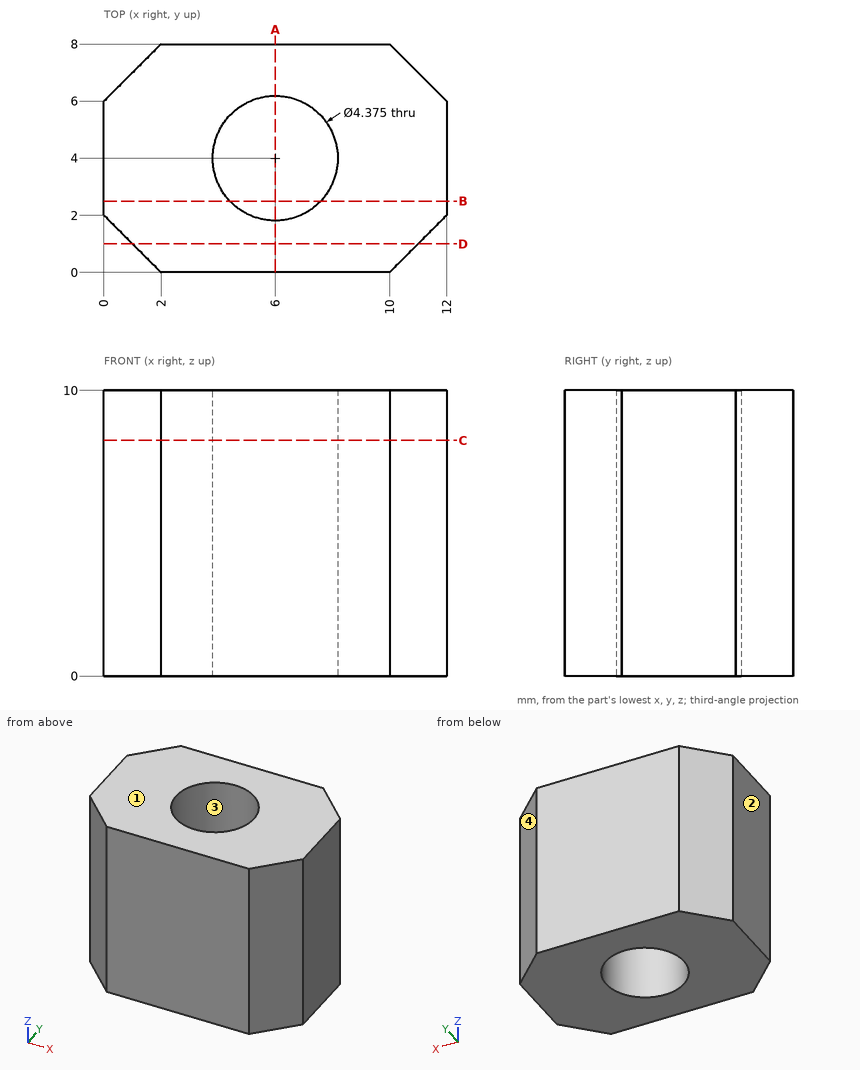
Can you work these out from the drawing? Everything is in mm from the part's minimum corner. Coordinates: 2 decimals unless noted, no trailing zeros. Loops run counter-clockwise (first coordinate to the right, second up) from the corner with the lowest first, then second, coordinate; pieces in that order, holes last.
1. Imagine slicing it at C-C, the plane z = 8.25. Please give me the cut outline in (x, y) (1 decimal), and give its area (3 significant figures).
2. If we mould it in two halves opening along X, with no side actions, what happens to the marked faces 1, 2, 3 and 4? For each: pulls with the +X half, pulls with the -X half, needs draft (parallel to the pull), parting line crosses it, or undercut.
3. Imagine slicing it at A-A, the plane x = 6. Please give me the cut outline in (y, z), and give its area (4 significant figures).
4. Imagine slicing it at D-D, the plane y = 1. Please give me the cut outline in (x, z).
5. I need wall thicknesses on L1, parallel to Y at x = 6, z = 2; L2, parallel to X at y = 3.5, z = 2.25; L3, parallel to Y at x = 7.25, z = 4.25. Which ranges of each line are inside material? Lowest first, please.
6. For P1, Ø4, axis at x = 6, y = 4, coming from the -Z side, with a flat end and sliding along its axis, tell me the tip position at first contact or that it passes through.
7. Imagine slicing it at B-B, the plane y = 2.5. Please give me the cut outline in (x, z).
Taken from the geometry:
1. outline: (0, 2) - (2, 0) - (10, 0) - (12, 2) - (12, 6) - (10, 8) - (2, 8) - (0, 6) - close; hole circle Ø4.4 at (6, 4)
1. area: 73.0 mm2
2. face 1: needs draft
2. face 2: pulls with the -X half
2. face 3: undercut
2. face 4: pulls with the +X half
3. outline: (0, 0) - (1.81, 0) - (1.81, 10) - (0, 10) - close; (6.19, 0) - (8, 0) - (8, 10) - (6.19, 10) - close
3. area: 36.25 mm2
4. outline: (1, 0) - (11, 0) - (11, 10) - (1, 10) - close
5. L1: y = 0 to 1.81, 6.19 to 8
5. L2: x = 0 to 3.87, 8.13 to 12
5. L3: y = 0 to 2.2, 5.8 to 8
6. P1: passes through
7. outline: (0, 0) - (4.41, 0) - (4.41, 10) - (0, 10) - close; (7.59, 0) - (12, 0) - (12, 10) - (7.59, 10) - close
